Can you work these out from the drawing? Everything is in mm from the part's minimum corner. Give positions to 0.01 mm unless a question says otherwise; leave off trailing zeros. Loops run counter-clockwise (first coordinate to the right, second up) from the corner with the lowest first, then second, coordinate; pieces in that order, holes last. Notation, with made-up numbers: (-27, 55.5) - (27, 55.5) arc R19 cw to (27, 86.5) - close; hole circle Ø6 at (-4, 8.25). An arc over 180 degrees is marked (long way). Answer in a Markdown table with one row per item.
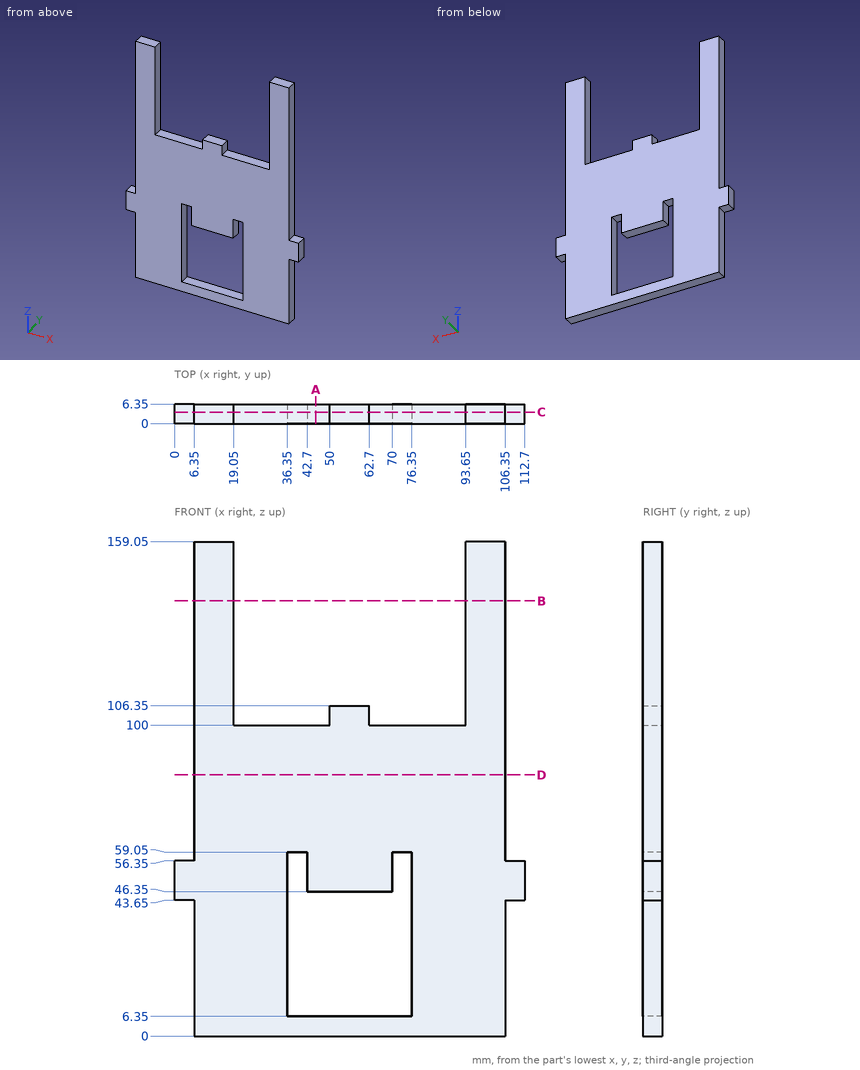
Q1. Imagine slicing it at A-A, the plane x = 45.5. Write out the boundary of the cut face in (y, z), and give its area (3 significant figures).
Checked values:
| item | result |
|---|---|
| outline | (0, 0) - (6.35, 0) - (6.35, 6.35) - (0, 6.35) - close; (0, 46.35) - (6.35, 46.35) - (6.35, 100) - (0, 100) - close |
| area | 381 mm² |
Q2. Imagine slicing it at B-B, the plane z = 140. Write out the boundary of the cut face in (x, y), and give its area (3 significant figures).
Checked values:
| item | result |
|---|---|
| outline | (6.35, 0) - (19.05, 0) - (19.05, 6.35) - (6.35, 6.35) - close; (93.65, 0) - (106.35, 0) - (106.35, 6.35) - (93.65, 6.35) - close |
| area | 161 mm² |
Q3. Imagine slicing it at D-D, the plane z = 84. Write out the boundary of the cut face in (x, y).
Checked values:
| item | result |
|---|---|
| outline | (6.35, 0) - (106.35, 0) - (106.35, 6.35) - (6.35, 6.35) - close |
Q4. If I drill on line 1 (X direction, y = 2.25, z = 10); line 2 (X direction, y = 3.75, z = 117.5); line 3 (Z direction, x = 57.5, y = 4.25), over which ranges is the centre line in solid material (lowest first)? Write a range as [from, to].
Checked values:
| item | result |
|---|---|
| line 1 | x = [6.35, 36.35], [76.35, 106.35] |
| line 2 | x = [6.35, 19.05], [93.65, 106.35] |
| line 3 | z = [0, 6.35], [46.35, 106.35] |
Q5. Imagine slicing it at C-C, the plane y = 3.75. Write out the boundary of the cut face in (x, z), and give its area (3 significant figures).
Checked values:
| item | result |
|---|---|
| outline | (0, 43.65) - (6.35, 43.65) - (6.35, 0) - (106.35, 0) - (106.35, 43.65) - (112.7, 43.65) - (112.7, 56.35) - (106.35, 56.35) - (106.35, 159.05) - (93.65, 159.05) - (93.65, 100) - (62.7, 100) - (62.7, 106.35) - (50, 106.35) - (50, 100) - (19.05, 100) - (19.05, 159.05) - (6.35, 159.05) - (6.35, 56.35) - (0, 56.35) - close; hole (36.35, 6.35) - (76.35, 6.35) - (76.35, 59.05) - (70, 59.05) - (70, 46.35) - (42.7, 46.35) - (42.7, 59.05) - (36.35, 59.05) - close |
| area | 9,980 mm² |
Q6. For pin 1 (2 mm diameter, centred on y = 4, z = 136, fed in from +X); pin 2 (2 mm diameter, centred on y = 1.5, z = 117.5, fed in from -X), each with a flat end and sliding along its axis, tell me the tip position at first contact or that it passes through.
Checked values:
| item | result |
|---|---|
| pin 1 | stops at x = 106.35 |
| pin 2 | stops at x = 6.35 |
